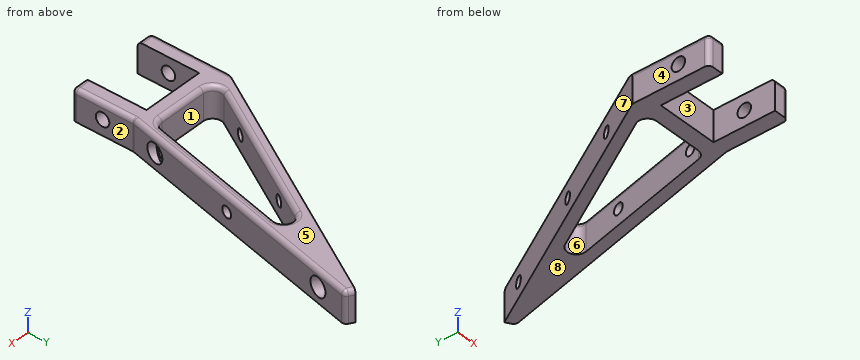
```python
from build123d import *

# Parameters (mm, degrees)
BOSS_EXTRUDE1_DEPTH = 10
CUT_EXTRUDE1_DEPTH  = 95.596978287
FILLET1_R           = 3
FILLET2_R           = 1.5
SKETCH3_R           = 2.2
CUT_EXTRUDE2_DEPTH  = 102.020680113
SKETCH4_R           = 1.75
CUT_EXTRUDE3_DEPTH  = 94.58236857
CUT_EXTRUDE4_START  = 3
SKETCH5_R           = 3
CUT_EXTRUDE4_DEPTH  = 91.712514751
CUT_EXTRUDE5_START  = -24.38
SKETCH6_R           = 3
CUT_EXTRUDE5_DEPTH  = 70.20236857


with BuildPart() as part:
    # Sketch1 → Boss-Extrude1 (new body)
    with BuildSketch(Plane.XY):
        Polygon((-10, -20), (-10, 0), (10, 0), (10, -20), (15, -20), (15, 0), (35.101483834, 85.770445967), (32.5, 87.27241336), (-15, 5), (-15, -20), align=None)
    extrude(amount=BOSS_EXTRUDE1_DEPTH)

    # Sketch2 → Cut-Extrude1 (cut, through all)
    with BuildSketch(Plane.XY.offset(10)):
        Polygon((-10.917498512, 5), (28.214788811, 72.779109859), (12.329822075, 5), align=None)
    extrude(amount=-CUT_EXTRUDE1_DEPTH, mode=Mode.SUBTRACT)

    # Fillet1
    fillet1_edges = [part.edges().sort_by_distance(p)[0] for p in [
        (28.214788811, 72.779109859, 5),
        (12.329822075, 5, 5),
        (-10.917498512, 5, 5),
    ]]
    fillet(fillet1_edges, radius=FILLET1_R)

    # Fillet2
    fillet2_edges = [part.edges().sort_by_distance(p)[0] for p in [
        (12.5, -20, 10),
        (-15, -20, 5),
        (35.101483834, 85.770445967, 5),
        (15, 0, 5),
        (15, -20, 5),
        (15, -10, 10),
        (25.050741917, 42.885222984, 10),
        (33.800741917, 86.521429663, 10),
        (-15, -7.5, 10),
        (-12.5, -20, 10),
        (4.871758353, 32.347795103, 10),
        (18.227176379, 30.163252268, 10),
        (2.115139497, 5, 10),
        (21.765145456, 56.485016027, 10),
        (11.815273588, 5.649082253, 10),
        (-8.3194223, 6.5, 10),
    ]]
    fillet(fillet2_edges, radius=FILLET2_R)

    # Sketch3 → Cut-Extrude2 (cut, through all)
    with BuildSketch(Plane.ZY.offset(15)):
        with Locations(Location((5, -10, 0), (0, 0, 270))):
            Circle(SKETCH3_R)
    extrude(amount=-CUT_EXTRUDE2_DEPTH, mode=Mode.SUBTRACT)

    # Sketch4 → Cut-Extrude3 (cut, through all)
    with BuildSketch(Plane(origin=(-13.415063509, 7.745190528, 0), x_dir=(0, 0, 1), z_dir=(-0.8660254037844382, 0.500000000000001, 0))):
        with Locations(Location((5, 81.330127019, 0), (0, 0, 270))):
            Circle(SKETCH4_R)
        with Locations(Location((5, 44.830127019, 0), (0, 0, 270))):
            Circle(SKETCH4_R)
        with Locations(Location((5, 16.098937019, 0), (0, 0, 270))):
            Circle(SKETCH4_R)
    extrude(amount=-CUT_EXTRUDE3_DEPTH, mode=Mode.SUBTRACT)

    # Sketch5 → Cut-Extrude4 (cut, through all)
    with BuildSketch(Plane(origin=(-13.480526942, 7.631804537, 0), x_dir=(0, 0, -1), z_dir=(0.866025403784438, -0.5000000000000009, 0)).offset(CUT_EXTRUDE4_START)):
        with Locations(Location((-5, 81.461053884, 0), (0, 0, 90))):
            Circle(SKETCH5_R)
    extrude(amount=CUT_EXTRUDE4_DEPTH, mode=Mode.SUBTRACT)

    # Sketch6 → Cut-Extrude5 (cut, through all)
    with BuildSketch(Plane(origin=(-13.415063509, 7.745190528, 0), x_dir=(0, 0, 1), z_dir=(-0.8660254037844382, 0.500000000000001, 0)).offset(CUT_EXTRUDE5_START)):
        with Locations(Location((5, 16.098937019, 0), (0, 0, 270))):
            Circle(SKETCH6_R)
    extrude(amount=-CUT_EXTRUDE5_DEPTH, mode=Mode.SUBTRACT)


solid = part.part
```
The model under review builds one solid part; all positions refer to its coordinate system, in mm. Face numbers are marked on the shaded views. A direction names the side the tool comes from. Give positions to 0.01 mm unless a question says otherwise; leave off trailing zeros. Write each loop counter-clockwise with the first axis right and the second up, starting at its lowest first coordinate (ties: lowest second). Pieces come first, ordered by that corner, then holes. Notation, with made-up numbers: (-1, 74.25) - (16, 74.25) arc R20 ccw to (16, 108.25) - close; hole circle Ø1 at (0, 41). An arc over 180 degrees is marked (long way). Answer in a Markdown table with one row per item. Add a question column.
1. Draft analysis for pull direction X (two halves, no side actions). For the marked faces 6, 7 and 8, state which applies: +X half, -X half, draft (parallel to the pull), parting line (faces both ways), or undercut.
2. Insertion check: P1, Ø2, axis at x = -8, z = 8.5, coming from the +Y side; P2, Ø5, axis at x = 5, z = 6, coming from the +Y side; P3, Ø4, axis at x = -3, z = 7, coming from the +Y side; P4, Ø2.5, axis at y = -10, z = 5, coming from the -X side. Each pin has a flat end and moves straight along its axis. Give the tip position at first contact, or say it passes through.
3. We need section A-A on y = -10. Write out the cut boundary in (x, z), then the cut area to 3 significant figures.
4. Wall thickness on line 1 along X through (y, z) = (-15, 6); line 2 along Z through (x, y) = (-12, -10); line 3 along X through (y, z) = (26, 4): over which ranges is each line inside the solid? List them lowest first. Write a range as [from, to].
5. We need section B-B on x = 22. State how many separate pieces and enclosed holes the cut face has, then the cut area to 3 significant figures.
6. Tool access review of the marked faces 1, 2, 3, 4 and 5: name each direction out of +Z, -Z, +X, -X, +Y, -Y from which nothing blocks a thin tool from reaching the whole face with its end or side.
Ans:
| question | item | result |
|---|---|---|
| 1 | face 6 | undercut |
| 1 | face 7 | -X half |
| 1 | face 8 | draft |
| 2 | P1 | stops at y = 18.86 |
| 2 | P2 | stops at y = 43.97 |
| 2 | P3 | stops at y = 29.25 |
| 2 | P4 | passes through |
| 3 | outline | (-15, 0) - (-10, 0) - (-10, 2.8) - (-15, 2.8) - close; (-15, 7.2) - (-10, 7.2) - (-10, 10) - (-13.5, 10) arc R1.5 ccw to (-15, 8.5) - close; (10, 0) - (15, 0) - (15, 2.8) - (10, 2.8) - close; (10, 7.2) - (15, 7.2) - (15, 8.5) arc R1.5 ccw to (13.5, 10) - (10, 10) - close |
| 3 | area | 55.0 mm^2 |
| 4 | line 1 | x = [-15, -10], [10, 15] |
| 4 | line 2 | z = [0, 2.8], [7.2, 10] |
| 4 | line 3 | x = [-2.88, 1.21], [17.25, 21.09] |
| 5 | separate pieces | 2 |
| 5 | enclosed holes | 1 |
| 5 | area | 275 mm^2 |
| 6 | face 1 | +Z, -Z |
| 6 | face 2 | +Z, -Z, +X, -Y |
| 6 | face 3 | +Z, -Z, -Y |
| 6 | face 4 | +Z, -Z, -X, +Y, -Y |
| 6 | face 5 | +Z, +X, -X, +Y, -Y |
